Autodesk Inventor part; units mm, degrees
ref_plane "YZ Plane" through (0, 0, 0) normal (1, 0, 0) x (0, 1, 0)
ref_plane "XZ Plane" through (0, 0, 0) normal (0, 1, 0) x (-1, 0, 0)
ref_plane "XY Plane" through (0, 0, 0) normal (0, 0, 1) x (1, 0, 0)
sketch "Skizze1" plane through (0, 0, 0) normal (0, 1, 0) x (-1, 0, 0)
  line L0 (14, -11.5) -> (-14, -11.5)
  line L1 (-14, -11.5) -> (-14, 11.5)
  line L2 (-14, 11.5) -> (14, 11.5)
  line L3 (14, 11.5) -> (14, -11.5)
  line L4 (0, -16.1) -> (0, 16.1)
  line L5 (-19.6, 0) -> (19.6, 0)
  point P0 (0, 0)
  dimension "d0" = 28
  dimension "d1" = 23
extrude "Extrusion1" add sketch "Skizze1" along normal mid plane 2
sketch "Skizze2" plane through (0, 1, 0) normal (0, 1, 0) x (1, 0, 0)
  circle A0 centre (-10, 7.5) radius 1.6
  circle A1 centre (-10, -7.5) radius 1.6
  circle A2 centre (10, 7.5) radius 1.6
  circle A3 centre (10, -7.5) radius 1.6
  line L0 (0, 16.1) -> (0, -16.1)
  line L1 (19.6, 0) -> (-19.6, 0)
  point P0 (0, 0)
  dimension "d4" = 3.2
  dimension "d5" = 3.2
  dimension "d6" = 3.2
  dimension "d7" = 3.2
  dimension "d8" = 20
  dimension "d9" = 20
  dimension "d10" = 15
  dimension "d11" = 15
  dimension "d12" = 7.5
  dimension "d13" = 10
  dimension "d14" = 10
  dimension "d15" = 7.5
extrude "Extrusion2" cut sketch "Skizze2" against normal up to surface (2 mm away)
properties part number "Ebene3_verbindung"
Source: CAD feature listing. Evaluate the final solid. Frame: model axes, mm. Coordinates: 2 decimals unless noted, no trailing zeros. Loops run counter-clockwise (first coordinate to the right, second up) from the corner with the lowest first, then second, coordinate; pieces in that order, holes last. Notation, with made-up numbers: M 15.5,-9 L 53.5,-9 A18 ccw 53.5,-5 Z; hole C 63,41.5 d11. An arc over 180 degrees is marked long. Put each result on its own line as item: value. Start each with the question number.
1) Contact query for a flat-ended pin moving along its axis: pin 1 Ø3 at (x, z) = (10, 7.5) entering from +Y. Output: stop coordinate, or through.
2) Cut plane C-C on x = 10. Return the cut outline in (y, z).
3) Cut plane A-A on z = 7.5. Return the cut outline in (x, y).
4) Ray query, L1, parallel to Z at x = 10, y = -0.3; L2, parallel to X at y = -0.5, z = 7.5; L3, parallel to Z at x = 9.25, y = 0.25. Return the intervals inside material, ascending. Write a range as from..to.
5) Cut plane B-B on y = -0.4. Return the cut outline in (x, z), then the cut area to 3 significant figures.
6) Pull-direction query (X, two-part tool) for faces 1 (the face through (0, 0, -11.5)), 2 (the face through (14, 0, 0)), 3 (the face through (-11.27, 0.01, 8.47)); classes: pulls with the +X half, pulls with the -X half, needs draft (parallel to the pull), parting line crosses it, or undercut.
The answers:
1. pin 1: passes through
2. outline: M -1,-11.5 L 1,-11.5 L 1,-9.1 L -1,-9.1 Z; M -1,-5.9 L 1,-5.9 L 1,5.9 L -1,5.9 Z; M -1,9.1 L 1,9.1 L 1,11.5 L -1,11.5 Z
3. outline: M -14,-1 L -11.6,-1 L -11.6,1 L -14,1 Z; M -8.4,-1 L 8.4,-1 L 8.4,1 L -8.4,1 Z; M 11.6,-1 L 14,-1 L 14,1 L 11.6,1 Z
4. L1: z = -11.5..-9.1, -5.9..5.9, 9.1..11.5
4. L2: x = -14..-11.6, -8.4..8.4, 11.6..14
4. L3: z = -11.5..-8.91, -6.09..6.09, 8.91..11.5
5. outline: M -14,-11.5 L 14,-11.5 L 14,11.5 L -14,11.5 Z; hole C -10,-7.5 d3.2; hole C -10,7.5 d3.2; hole C 10,-7.5 d3.2; hole C 10,7.5 d3.2
5. area: 612 mm²
6. face 1: needs draft
6. face 2: pulls with the +X half
6. face 3: undercut
